```python
from build123d import *

# Parameters (mm, degrees)
SKETCH1_R           = 25
BOSS_EXTRUDE1_DEPTH = 25
SKETCH2_R           = 17.5
CUT_EXTRUDE1_DEPTH  = 3
SKETCH3_R           = 20
BOSS_EXTRUDE2_DEPTH = 40
SKETCH4_R           = 17.5
BOSS_EXTRUDE3_DEPTH = 3
FILLET1_R           = 3


with BuildPart() as part:
    # Sketch1 → Boss-Extrude1 (new body, symmetric)
    with BuildSketch(Plane.XY):
        Circle(SKETCH1_R)
    extrude(amount=BOSS_EXTRUDE1_DEPTH, both=True)

    # Sketch2 → Cut-Extrude1 (cut)
    with BuildSketch(Plane.XY.offset(25)):
        Circle(SKETCH2_R)
    cut_extrude1 = extrude(amount=-CUT_EXTRUDE1_DEPTH, mode=Mode.SUBTRACT)

    # Mirror1: Cut-Extrude1 across plane
    add(cut_extrude1.mirror(Plane.XY), mode=Mode.SUBTRACT)

    # Sketch3 → Boss-Extrude2 (add)
    with BuildSketch(Plane(origin=(0, 0, 0), x_dir=(0, 0, -1), z_dir=(1, 0, 0))):
        Circle(SKETCH3_R)
    extrude(amount=BOSS_EXTRUDE2_DEPTH)

    # Sketch4 → Boss-Extrude3 (add)
    with BuildSketch(Plane(origin=(40, 0, 0), x_dir=(0, 0, -1), z_dir=(1, 0, 0))):
        Circle(SKETCH4_R)
    extrude(amount=BOSS_EXTRUDE3_DEPTH)

    # Fillet1
    fillet1_edges = [part.edges().sort_by_distance(p)[0] for p in [
        (15, 20, 0),
    ]]
    fillet(fillet1_edges, radius=FILLET1_R)


solid = part.part
```
Check sheet for the modelled part. Datum: model origin and axes. Units: mm. A direction names the side the tool comes from. Give positions to 0.01 mm unless a question says otherwise; leave off trailing zeros. Order: outer loops, then holes, each group sorted by start corner. A loop starts at its lowest first (then second) coordinate and runs counter-clockwise, first axis right, second up. Notation, with made-up numbers: (-31.75, 47.5) -> (-3.75, 47.5) arc R19 cw to (-3.75, 71.5) -> close; hole circle Ø9 at (-27, 72.25). An arc over 180 degrees is marked (long way). Use CSV: the item, a comma, the result in double quotes. Start each with the question number.
1) Sectioned sample at A-A, the plane x = 0. Record the boundary of the cut face in (y, z), plus the area to 3 significant figures.
2) Mould release check, pull along X, two halves, no side actions. Record for faces 1 (the face through (41.479, -10.648, 13.887)), 2 (the face through (-13.887, -10.648, -23.521)), 3 (the face through (43, 0, 0)): released by +X, released by -X, zero draft, split by the parting line, or undercut.
3) Material ranges on line 1 (Y direction, x = 0, z = 23); line 2 (Z direction, x = 3, y = 15.5); line 3 (X direction, y = 19, z = 7), recorded low to high. Write a range as from..to.
4) Sectioned sample at C-C, the plane x = 29.5. Record the boundary of the cut face in (y, z).
5) Sectioned sample at B-B, the plane x = -9.5. Record the boundary of the cut face in (y, z), plus the area to 3 significant figures.
6) Set-up check for faces 4 (the face through (-17, -5, 25)), 5 (the face through (40, -18, 0)), 6 (the face through (0, 0, -22)), 7 (the face through (0, 0, 22)): record each of +Z, -Z, +X, -X, +Y, -Y from which the full face is reachable in a straight line by a thin tool's end or side.
7) Go/stop test with flat-tipped pins: P1, Ø6, axis at y = 8.5, z = 9, coming from the -X side; P2, Ø6, axis at y = 18.5, z = 15, coming from the +X side; P3, Ø6, axis at x = 1, z = -9.5, coming from the -Y side. Record where each tip stops, or that it passes through.
Recorded:
1,outline,"(-25, -25) -> (-17.5, -25) -> (-17.5, -22) -> (17.5, -22) -> (17.5, -25) -> (25, -25) -> (25, 25) -> (17.5, 25) -> (17.5, 22) -> (-17.5, 22) -> (-17.5, 25) -> (-25, 25) -> close"
1,area,"2,290 mm2"
2,face 1,"zero draft"
2,face 2,"undercut"
2,face 3,"released by +X"
3,line 1,"-25..-17.5, 17.5..25"
3,line 2,"-22..22"
3,line 3,"-16.25..16.53"
4,outline,"circle Ø40 at (0, 0)"
5,outline,"(-23.12, -25) -> (-14.7, -25) -> (-14.7, -22) -> (14.7, -22) -> (14.7, -25) -> (23.12, -25) -> (23.12, 25) -> (14.7, 25) -> (14.7, 22) -> (-14.7, 22) -> (-14.7, 25) -> (-23.12, 25) -> close"
5,area,"2,140 mm2"
6,face 4,"+Z, +X, -X, +Y, -Y"
6,face 5,"+X"
6,face 6,"-Z"
6,face 7,"+Z"
7,P1,"x = -24.39"
7,P2,"x = 19.62"
7,P3,"y = -25"
